Here's how the part is built. I have some questions about the finished solid (model axes, mm). A direction names the side the tool comes from. Coordinates: 2 decimals unless noted, no trailing zeros. Write each loop counter-clockwise with the first axis right and the second up, starting at its lowest first coordinate (ties: lowest second). Pieces come first, ordered by that corner, then holes.
```python
from build123d import *

# Parameters (mm, degrees)
SKETCH1_W           = 10
SKETCH1_H           = 10
BOSS_EXTRUDE1_DEPTH = 20
SKETCH1_3_W         = 10
SKETCH1_3_H         = 10
BOSS_EXTRUDE2_DEPTH = 20
SKETCH1_4_W         = 10
SKETCH1_4_H         = 40
BOSS_EXTRUDE3_DEPTH = 20
SKETCH1_5_W         = 10
SKETCH1_5_H         = 10
BOSS_EXTRUDE4_DEPTH = 50
SKETCH1_6_W         = 30
SKETCH1_6_H         = 10
BOSS_EXTRUDE5_DEPTH = 10
CHAMFER1_SIZE2      = 39.991364166
CHAMFER1_SIZE       = 20
FILLET1_R           = 10
SKETCH1_7_W         = 10
SKETCH1_7_H         = 40
SKETCH1_7_H_2       = 10
SKETCH1_7_W_2       = 30
BOSS_EXTRUDE6_DEPTH = 10


with BuildPart() as part:
    # Sketch1 → Boss-Extrude1 (new body)
    with BuildSketch(Plane(origin=(0, 0, 0), x_dir=(1, 0, 0), z_dir=(0, 1, 0))):
        with Locations((-47.852369013, 15)):
            Rectangle(SKETCH1_W, SKETCH1_H)
    extrude(amount=BOSS_EXTRUDE1_DEPTH)

    # Sketch1<3> → Boss-Extrude2 (add)
    with BuildSketch(Plane(origin=(0, 0, 0), x_dir=(1, 0, 0), z_dir=(0, 1, 0))):
        with Locations((-37.852369013, 15)):
            Rectangle(SKETCH1_3_W, SKETCH1_3_H)
    extrude(amount=BOSS_EXTRUDE2_DEPTH)

    # Sketch1<4> → Boss-Extrude3 (add)
    with BuildSketch(Plane(origin=(0, 0, 0), x_dir=(1, 0, 0), z_dir=(0, 1, 0))):
        with Locations((-47.852369013, -10)):
            Rectangle(SKETCH1_4_W, SKETCH1_4_H)
    extrude(amount=BOSS_EXTRUDE3_DEPTH)



with BuildPart() as body_2:
    # Sketch1<5> → Boss-Extrude4 (new body)
    with BuildSketch(Plane(origin=(0, 0, 0), x_dir=(1, 0, 0), z_dir=(0, 1, 0))):
        with Locations((2.147630987, 15)):
            Rectangle(SKETCH1_5_W, SKETCH1_5_H)
    extrude(amount=BOSS_EXTRUDE4_DEPTH)


with BuildPart() as part_1:
    add(part.part)

    add(body_2.part)  # Boss-Extrude5 merges body 2
    # Sketch1<6> → Boss-Extrude5 (add)
    with BuildSketch(Plane(origin=(0, 0, 0), x_dir=(1, 0, 0), z_dir=(0, 1, 0))):
        with Locations((-17.852369013, 15)):
            Rectangle(SKETCH1_6_W, SKETCH1_6_H)
    extrude(amount=BOSS_EXTRUDE5_DEPTH)

    # Chamfer1
    chamfer1_edges = [part_1.edges().sort_by_distance(p)[0] for p in [
        (-47.852369013, 20, 30),
    ]]
    chamfer1_side = [part_1.faces().sort_by_distance(p)[0] for p in [
        (-47.852369013, 19.6, 30),
    ]]
    chamfer(chamfer1_edges, length=CHAMFER1_SIZE - 0.0001, length2=CHAMFER1_SIZE2 - 0.0001, reference=chamfer1_side[0])  # a hair under: the kernel refuses the full size

    # Fillet1
    fillet1_edges = [part_1.edges().sort_by_distance(p)[0] for p in [
        (7.147630987, 50, -15),
    ]]
    fillet(fillet1_edges, radius=FILLET1_R - 0.0001)  # a hair under: the kernel refuses the full size

    # Sketch1<7> → Boss-Extrude6 (add)
    with BuildSketch(Plane(origin=(0, 0, 0), x_dir=(1, 0, 0), z_dir=(0, 1, 0))):
        with Locations((-47.852369013, -10)):
            Rectangle(SKETCH1_7_W, SKETCH1_7_H)
        with BuildLine():
            Line((-42.852369013, 10), (-42.852369013, -30))
            Line((-42.852369013, -30), (-32.852369013, -30))
            ThreePointArc((-32.852369013, -30), (-25.781301201, -27.071067812), (-22.852369013, -20))
            Line((-22.852369013, -20), (-22.852369013, 0))
            Line((-22.852369013, 0), (-2.852369013, 0))
            ThreePointArc((-2.852369013, 0), (4.218698799, 2.928932188), (7.147630987, 10))
            Line((7.147630987, 10), (-2.852369013, 10))
            Line((-2.852369013, 10), (-32.852369013, 10))
            Line((-32.852369013, 10), (-42.852369013, 10))
        make_face()
        with Locations((-47.852369013, 15)):
            Rectangle(SKETCH1_7_W, SKETCH1_7_H_2)
        with Locations((-37.852369013, 15)):
            Rectangle(SKETCH1_7_W, SKETCH1_7_H_2)
        with Locations((-17.852369013, 15)):
            Rectangle(SKETCH1_7_W_2, SKETCH1_7_H_2)
        with Locations((2.147630987, 15)):
            Rectangle(SKETCH1_7_W, SKETCH1_7_H_2)
    extrude(amount=-BOSS_EXTRUDE6_DEPTH)


solid = part_1.part
```
1) Imagine slicing it at A-A on x = -34.5. Please give me the cut outline in (y, z), then the cut area to 3 significant figures.
Values follow:
outline: (-10, -20) - (20, -20) - (20, -10) - (0, -10) - (0, 30) - (-10, 30) - close
area: 700 mm2
2) Imagine slicing it at B-B on y = 18. Please give me the cut outline in (x, z), then the cut area to 3 significant figures.
Values follow:
outline: (-52.85, -20) - (-32.85, -20) - (-32.85, -10) - (-42.85, -10) - (-42.85, -5.99) - (-52.85, -5.99) - close; (-2.85, -20) - (7.15, -20) - (7.15, -10) - (-2.85, -10) - close
area: 340 mm2
3) I need wall thicknesses on probe 1 along Y at (x, z) = (-32, 5); probe 2 along X at (y, z) = (5, -5); probe 3 along X at (y, z) = (43, -15.5). Which ranges of each line are inside material? Lowest first, please.
Values follow:
probe 1: y = -10 to 0
probe 2: x = -52.85 to -42.85
probe 3: x = -2.85 to 6.69
4) On a 3-axis mill with a long thin cutter (end or side, diameter ignored), from which of +Z, -Z, +X, -X, +Y, -Y can I reach the whole of each face in a straight line? I mean faces 1 (the face through (-13, 8, -10)), 2 (the face through (-43, 20, -15)), 3 (the face through (-22.852, -5, 10)), 4 (the face through (-30, -10, -1)), 5 (the face through (-32.852, 15, -15)). Say none if no direction works.
Values follow:
face 1: +Z, +X, +Y
face 2: +Z, -Z, -X, +Y
face 3: +Z, +X, +Y, -Y
face 4: +Z, -Z, +X, -X, -Y
face 5: +Z, -Z, +Y
5) Will these pins go through, and if not, where does the flat tip stop? pin 1 (3 mm diameter, centred on x = -18, z = -13.5, fed in from +Y); pin 2 (20 mm diameter, centred on x = -11, z = 16, fed in from +Y); pin 3 (3 mm diameter, centred on y = -7.5, z = 6, fed in from +X); pin 4 (8 mm diameter, centred on x = -10, y = -3.5, fed in from +Z).
Values follow:
pin 1: stops at y = 10
pin 2: passes through
pin 3: stops at x = -22.85
pin 4: stops at z = 0
6) We'd pull the mould along X, two halves only. Please class faces 6 (the face through (-13, -5, 0)), 7 (the face through (4.14, -4.93, -2.85)), 8 (the face through (-2.852, 30, -15)), 9 (the face through (-52.852, 2, -1)): pulls with the +X half, pulls with the -X half, needs draft (parallel to the pull), parting line crosses it, or undercut.
Values follow:
face 6: needs draft
face 7: pulls with the +X half
face 8: undercut
face 9: pulls with the -X half
7) Imagine slicing it at D-D on y = 7.5. Please give me the cut outline in (x, z).
Values follow:
outline: (-52.85, -20) - (7.15, -20) - (7.15, -10) - (-42.85, -10) - (-42.85, 15) - (-52.85, 15) - close
